Can you work these out from the model? Positions are in its coordinate system, mm. A direction names the side the tool comes from. Coordinates: 2 decimals unless noted, no trailing zeros. Order: outer loops, then holes, each group sorted by start corner. A loop starts at its lowest first (then second) coordinate and runs counter-clockwise, first axis right, second up. Notation, with made-up numbers: (-38, 86) -> (-15, 86) arc R29 ccw to (-15, 116) -> close; hole circle Ø4 at (-34.5, 63.5). An arc over 180 degrees is marked (long way). Answer as a JSON object with one key per item and string values. Group by question number.
(1) For pin 1 (2 mm diameter, centred on y = -27, z = 1.5, fed in from -X); pin 2 (6 mm diameter, centred on x = 5, y = 12.5, fed in from -Z); pin 3 (1.2 mm diameter, centred on x = -51.5, z = 1.5, fed in from +Y), each with a flat end and sliding along its axis, tell me the tip position at first contact or that it passes through.
(2) I want a section at B-B, the plane x = 35. List the corners of the cut face in (y, z) for me.
(3) If we mould it in two halves opening along Y, with no side actions, what happens to faces 4 (the flat face through (-52, 15, 2)), 5 (the flat face through (50, 27, 2)), 6 (the flat face through (0, 34, 2))? For each: pulls with the +Y half, pulls with the -Y half, needs draft (parallel to the pull), parting line crosses it, or undercut.
(4) I need wall thicknesses on line 1 (Y direction, x = 38.5, z = 0.3); line 2 (X direction, y = 25.5, z = 2.6). Which ranges of each line are inside material? Lowest first, please.
(5) Which directions (+Z, -Z, +X, -X, +Y, -Y) give clear straight access to the entire face, cutting with the end or side of a thin tool? Please do faces 1 (the flat face through (-50, 28, 2)), 2 (the flat face through (50, -28, 2)), 3 (the flat face through (-50, -27, 2)).
from build123d import *

# Parameters (mm, degrees)
BOSS_EXTRUDE1_DEPTH = 4
SKETCH2_W           = 20
SKETCH2_H           = 8
BOSS_EXTRUDE2_DEPTH = 4


with BuildPart() as part:
    # Sketch1 → Boss-Extrude1 (new body)
    with BuildSketch(Plane.XY):
        Polygon((-50, 30), (-50, 25), (-54, 25), (-54, 15), (-50, 15), (-50, 5), (-54, 5), (-54, -5), (-50, -5), (-50, -15), (-54, -15), (-54, -25), (-50, -25), (-50, -30), (50, -30), (50, -25), (54, -25), (54, -15), (50, -15), (50, -5), (54, -5), (54, 5), (50, 5), (50, 15), (54, 15), (54, 25), (50, 25), (50, 30), align=None)
    extrude(amount=BOSS_EXTRUDE1_DEPTH)

    # Sketch2 → Boss-Extrude2 (add)
    with BuildSketch(Plane.XY.offset(4)):
        with Locations((0, 30)):
            Rectangle(SKETCH2_W, SKETCH2_H)
    extrude(amount=-BOSS_EXTRUDE2_DEPTH)


solid = part.part
Computed values:
{
 "1": {"pin 1": "stops at x = -50", "pin 2": "stops at z = 0", "pin 3": "stops at y = 25"},
 "2": {"outline": "(-30, 0) -> (30, 0) -> (30, 4) -> (-30, 4) -> close"},
 "3": {"face 4": "undercut", "face 5": "needs draft", "face 6": "pulls with the +Y half"},
 "4": {"line 1": "y = -30 to 30", "line 2": "x = -50 to 50"},
 "5": {"face 1": "+Z, -Z, -X, +Y", "face 2": "+Z, -Z, +X, -Y", "face 3": "+Z, -Z, -X, -Y"}
}
